Print and shaded views of the part. All mm, measured from the part's lowest x, y and z. A direction names the side the tool comes from. Round coordinates to 2 decimals unless told otherwise and drop trailing zeros. Order: outer loops, then holes, each group sorted by start corner. A loop starts at its lowest first (then second) coordinate and runs counter-clockwise, first axis right, second up. Notation, with made-up numbers: (11.5, 88.5) - (31.5, 88.5) arc R9 cw to (31.5, 100.5) - close; hole circle Ø9 at (-7.75, 49). An arc over 180 degrees is marked (long way). Return JSON: item names as keys, results as strings. Group by question number.
Item 1: Saw through at A-A on z = 50.5. List the corners of the cut face in (x, y).
Item 2: Saw through at C-C on x = 30.5. List the corners of the cut face in (y, z).
Item 3: Probe probe 1 along Y at (x, z) = (20.5, 21.5); probe 2 along X at (y, z) = (57, 9); probe 3 along Z at (x, y) = (122.5, 43). List the from-to ranges inside material, lowest first.
Item 4: Drop a flat-ended pin along its axis: pin 1 (1.5 mm diameter, centred on x = 120, y = 109, fed in from -Z). Give the stop position or say it passes through.
Item 5: Saw through at B-B on y = 94. List the corners of the cut face in (x, z).
Item 6: Two-plate mould, pull along Y, no slides. Class the marked faces 1, 2, 3 and 4: released by +Y, released by -Y, zero draft, split by the parting line, or undercut.
Item 7: Tool access for the marked faces 5 and 6: list every direction of +Z, -Z, +X, -X, +Y, -Y with a clear straight run to the whole face (end or side of a thin tool).
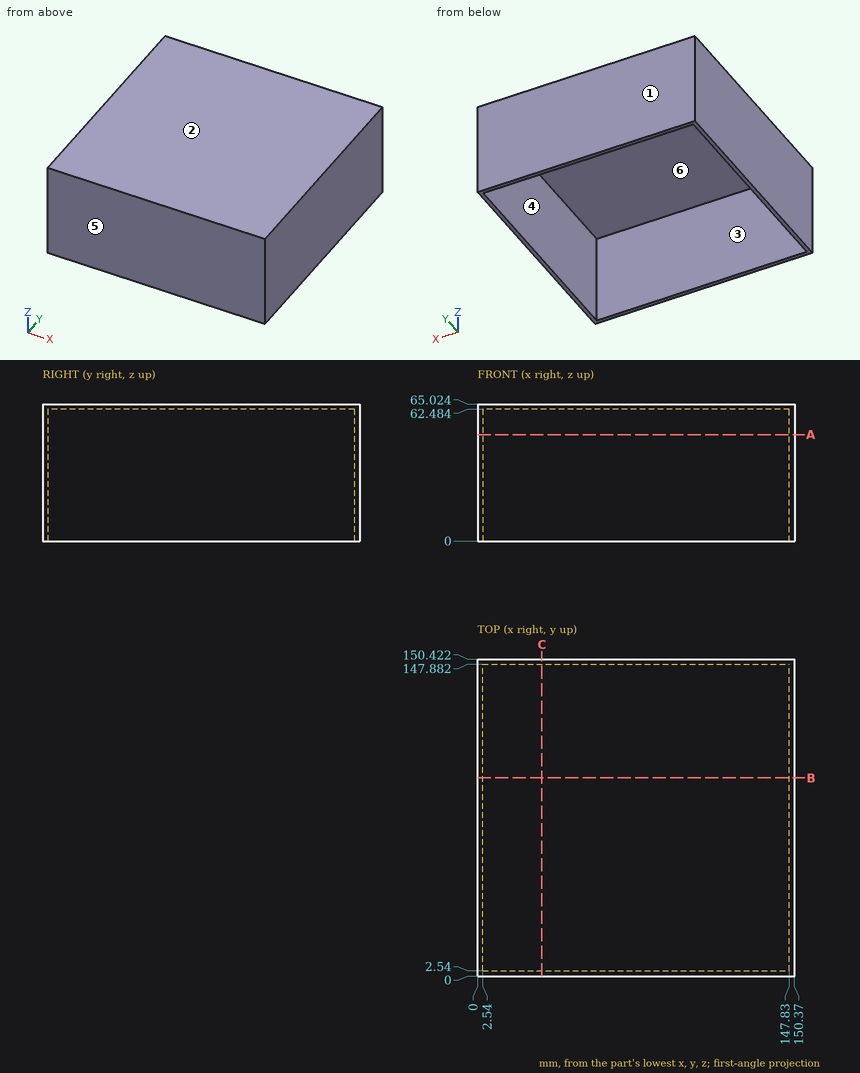
Filled in:
{
 "1": {"outline": "(0, 0) - (150.37, 0) - (150.37, 150.42) - (0, 150.42) - close; hole (2.54, 2.54) - (147.83, 2.54) - (147.83, 147.88) - (2.54, 147.88) - close"},
 "2": {"outline": "(0, 0) - (2.54, 0) - (2.54, 62.48) - (147.88, 62.48) - (147.88, 0) - (150.42, 0) - (150.42, 65.02) - (0, 65.02) - close"},
 "3": {"probe 1": "y = 0 to 2.54, 147.88 to 150.42", "probe 2": "x = 0 to 2.54, 147.83 to 150.37", "probe 3": "z = 62.48 to 65.02"},
 "4": {"pin 1": "stops at z = 62.48"},
 "5": {"outline": "(0, 0) - (2.54, 0) - (2.54, 62.48) - (147.83, 62.48) - (147.83, 0) - (150.37, 0) - (150.37, 65.02) - (0, 65.02) - close"},
 "6": {"face 1": "released by +Y", "face 2": "zero draft", "face 3": "undercut", "face 4": "undercut"},
 "7": {"face 5": "+Z, -Z, +X, -X, -Y", "face 6": "-Z"}
}
